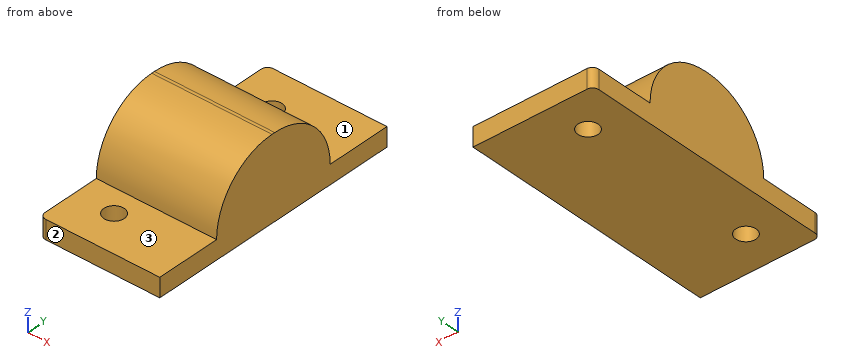
from build123d import *

# Parameters (mm, degrees)
F0_W     = 19
F0_H     = 41
F0_R     = 1.6
F1_DEPTH = 3
F2_R     = 1
F3_W     = 19
F3_H     = 20.5
F4_DEPTH = 10
F5_R     = 9.99999


# Not quite as in the source:
# - a fillet or chamfer is up to 0.001 mm smaller than in the source, because OpenCascade refuses the exact size


with BuildPart() as f1:
    # F0 (on Top) → F1 (new body)
    with BuildSketch(Plane.XY):
        with Locations((-9.5, 0)):
            Rectangle(F0_W, F0_H)
        with Locations((-12.7, -14.25)):
            Circle(F0_R, mode=Mode.SUBTRACT)
        with Locations((-12.7, 14.25)):
            Circle(F0_R, mode=Mode.SUBTRACT)
    extrude(amount=F1_DEPTH)

    # F2
    f2_edges = [f1.edges().sort_by_distance(p)[0] for p in [
        (-19, -20.5, 1.5),
        (-19, 20.5, 1.5),
    ]]
    fillet(f2_edges, radius=F2_R)

    # F3 (on face) → F4 (join)
    with BuildSketch(Plane.XY.offset(3)):
        with Locations((-9.5, 0)):
            Rectangle(F3_W, F3_H)
    extrude(amount=F4_DEPTH)

    # F5 (radius 10 in the source; OpenCascade refuses exactly that, so slightly less here)
    f5_edges = [f1.edges().sort_by_distance(p)[0] for p in [
        (-9.5, 10.25, 13),
        (-9.5, -10.25, 13),
    ]]
    fillet(f5_edges, radius=F5_R)


solid = f1.part
Verification items for the finished model (mm, model axes). Face numbers are marked on the shaded views. A direction names the side the tool comes from. Round coordinates to 2 decimals unless told otherwise and drop trailing zeros. Loops run counter-clockwise (first coordinate to the right, second up) from the corner with the lowest first, then second, coordinate; pieces in that order, holes last. Notation, with made-up numbers: (13, 44.25) - (65, 44.25) arc R21 ccw to (65, 57.25) - close; hole circle Ø4 at (28.5, -35.5). An arc over 180 degrees is marked (long way). Use a Markdown table: item, result. Add a question column.
1. Access from +Z, -Z, +X, -X, +Y, -Y to the whole of each face (thin tool, end or side, straight path). Record for the marked faces 1, 2 and 3.
2. Section check A-A, the plane y = -14.25. Record the boundary of the cut face in (x, z), plus the area to 3 significant figures.
3. Section check B-B, the plane x = -12.7. Give the number of separate pieces and of enclosed holes in the cut face, plus the area to 3 significant figures.
4. Section check D-D, the plane y = 17. Record the boundary of the cut face in (x, z), plus the area to 3 significant figures.
5. Gauge pin test, flat ends, axial feed: pin 1 (3 mm diameter, centred on y = 4.5, z = 4, fed in from +X); pin 2 (6 mm diameter, centred on x = -11.5, z = 10.5, fed in from -Y); pin 3 (3 mm diameter, centred on x = -12, y = 17, fed in from +Z); pin 4 (8 mm diameter, centred on x = -13, y = -13.5, fed in from +Z). Record the tip position at first contact, or that the pin passes through.
6. Thickness scan on probe 1 along Y at (x, z) = (-12.7, 1.5); probe 2 along Y at (x, z) = (-11.5, 2.5); probe 3 along Z at (x, y) = (-11.75, 12.5). Record the ranges inside material, lowest first. Write a range as [from, to].
Checks:
| question | item | result |
|---|---|---|
| 1 | face 1 | +Z, +X, -X, +Y |
| 1 | face 2 | +Z, -Z, +X, -X, -Y |
| 1 | face 3 | +Z, +X, -X, -Y |
| 2 | outline | (-19, 0) - (-14.3, 0) - (-14.3, 3) - (-19, 3) - close; (-11.1, 0) - (0, 0) - (0, 3) - (-11.1, 3) - close |
| 2 | area | 47.4 mm^2 |
| 3 | separate pieces | 3 |
| 3 | enclosed holes | 0 |
| 3 | area | 266 mm^2 |
| 4 | outline | (-19, 0) - (0, 0) - (0, 3) - (-19, 3) - close |
| 4 | area | 57.0 mm^2 |
| 5 | pin 1 | stops at x = 0 |
| 5 | pin 2 | stops at y = -9.18 |
| 5 | pin 3 | stops at z = 3 |
| 5 | pin 4 | stops at z = 6.8 |
| 6 | probe 1 | y = [-20.5, -15.85], [-12.65, 12.65], [15.85, 20.5] |
| 6 | probe 2 | y = [-20.5, -15.31], [-13.19, 13.19], [15.31, 20.5] |
| 6 | probe 3 | z = [0, 3] |
